The listing builds one solid part. Answer for the finished solid, in the listing's coordinates (mm). A direction names the side the tool comes from. Give positions to 0.01 mm unless a question says otherwise; leave off trailing zeros. Write each loop counter-clockwise with the first axis right and the second up, starting at its lowest first coordinate (ties: lowest second). Pieces come first, ordered by that corner, then holes. Notation, with made-up numbers: M 37,-10 L 41,-10 A14 ccw 41,-6 Z; hole C 36,38.25 d11. An arc over 180 degrees is marked long. Return JSON: item names as keys, results as strings.
from build123d import *

# Parameters (mm, degrees)
F1_DEPTH = 3.81
F2_R     = 6.35
F3_W     = 19.05
F3_H     = 44.45
F4_DEPTH = 3.81
F5_R     = 7.62
F6_R     = 1.905
F6_R_2   = 1.9053216062
F7_DEPTH = 25.4


# Not quite as in the source:
# - a feature names something its author has since deleted; it is built from what else it names


with BuildPart() as f1:
    # F0 (on Front) → F1 (new body)
    with BuildSketch(Plane.XZ):
        with BuildLine():
            Line((0, 19.1190056503), (0, 0))
            Line((0, 0), (19.05, 0))
            Line((19.05, 0), (19.05, 19.6883492172))
            ThreePointArc((19.05, 19.6883492172), (9.4277487791, 22.6576630171), (0, 19.1190056503))
        make_face()
    extrude(amount=F1_DEPTH)

    # F2
    f2_edges = [f1.edges().sort_by_distance(p)[0] for p in [
        (0, -1.905, 19.119006),
        (19.05, -1.905, 19.688349),
    ]]
    fillet(f2_edges, radius=F2_R)

    # F3 (on face) → F4 (join)
    with BuildSketch(Plane(origin=(0, 0, 0), x_dir=(1, 0, 0), z_dir=(0, 0, -1))):
        with Locations((9.525, 1.905)):
            Rectangle(F3_W, F3_H)
    extrude(amount=F4_DEPTH)

    # F5
    f5_edges = [f1.edges().sort_by_distance(p)[0] for p in [
        (19.05, -24.13, -1.905),
        (0, -24.13, -1.905),
        (19.05, 20.32, -1.905),
        (0, 20.32, -1.905),
    ]]
    fillet(f5_edges, radius=F5_R)

    # F6 (on face) → F7 (cut)
    with BuildSketch(Plane.XY):
        with Locations((9.525, 7.3555377312)):
            Circle(F6_R)
        with Locations((9.525, -10.8990902081)):
            Circle(F6_R_2)
    extrude(amount=-F7_DEPTH, mode=Mode.SUBTRACT)


solid = f1.part
Item 1: Find the intervals of material crossed by line 1 (Y direction, x = 3.75, z = 1); line 2 (Y direction, x = 13.5, z = -0.75), in increasing order.
Geometry results:
{"line 1": "y = -3.81 to 0", "line 2": "y = -23.84 to 20.03"}
Item 2: A cutting plane is placed at D-D, the plane x = 9.5. Write down the section's boundary in (y, z), plus the area to 3 significant figures.
Geometry results:
{"outline": "M -24.13,-3.81 L -12.8,-3.81 L -12.8,0 L -24.13,0 Z; M -8.99,-3.81 L 5.45,-3.81 L 5.45,0 L 0,0 L 0,22.66 L -3.81,22.66 L -3.81,0 L -8.99,0 Z; M 9.26,-3.81 L 20.32,-3.81 L 20.32,0 L 9.26,0 Z", "area": "227 mm2"}
Item 3: A cutting plane is placed at A-A, the plane y = 8. Write down the section's boundary in (x, z), plus the area to 3 significant figures.
Geometry results:
{"outline": "M 0,-3.81 L 7.73,-3.81 L 7.73,0 L 0,0 Z; M 11.32,-3.81 L 19.05,-3.81 L 19.05,0 L 11.32,0 Z", "area": "58.9 mm2"}
Item 4: A cutting plane is placed at C-C, the plane x = 1.5. Write down the section's boundary in (y, z), plus the area to 3 significant figures.
Geometry results:
{"outline": "M -21.05,-3.81 L 17.24,-3.81 L 17.24,0 L 0,0 L 0,19.71 L -3.81,19.71 L -3.81,0 L -21.05,0 Z", "area": "221 mm2"}
Item 5: Given pin 1 Ø6 at (x, y) = (9.52, 7.36) entering from -Z; pin 2 Ø5 at (x, z) = (13, 19) entering from -Y; pin 3 Ø2 at (x, z) = (3, 9) entering from +Y; pin 4 Ø9.5 at (x, y) = (5, 7.5) entering from +Z, each flat-ended and moving along its own axis, determine where each tip first touches the part or whether it passes through.
Geometry results:
{"pin 1": "stops at z = -3.81", "pin 2": "stops at y = -3.81", "pin 3": "stops at y = 0", "pin 4": "stops at z = 0"}
Item 6: Which of the six approach directions +Z, -Z, +X, -X, +Y, -Y give full straight-line access (tool end or side, diameter ignored) to faces 1 (the cylindrical face through (9.28, -9.01, -1.88)), 2 (the flat face through (9, 10, 0)), 3 (the flat face through (9, -14, 0))?
Geometry results:
{"face 1": "+Z, -Z", "face 2": "+Z, +X, -X, +Y", "face 3": "+Z, +X, -X, -Y"}
Item 7: A cutting plane is placed at B-B, the plane z = -1.25. Write down the section's boundary in (x, y) (3 decimals), plus the area to 3 significant figures.
Geometry results:
{"outline": "M 0,-16.51 A7.62 ccw 7.62,-24.13 L 11.43,-24.13 A7.62 ccw 19.05,-16.51 L 19.05,12.7 A7.62 ccw 11.43,20.32 L 7.62,20.32 A7.62 ccw 0,12.7 Z; hole C 9.525,-10.899 d3.811; hole C 9.525,7.356 d3.81", "area": "774 mm2"}
Item 8: Determine the mould class of faces 4 (the cylindrical face through (16.759, -21.957, -1.932)), 5 (the cylindrical face through (2.173, 18.029, -1.932)), 6 (the flat face through (9, -3.81, 11)), 7 (the cylindrical face through (8.12, 8.64, -1.88)) for opening direction X: +X half, -X half, draft (parallel to the pull), parting line (faces both ways), or undercut.
Geometry results:
{"face 4": "+X half", "face 5": "-X half", "face 6": "draft", "face 7": "undercut"}
